```python
from build123d import *

# Parameters (mm, degrees)
SKETCH1_R           = 28
SKETCH1_R_2         = 18
BOSS_EXTRUDE1_DEPTH = 22
SKETCH2_W           = 56
SKETCH2_H           = 56
BOSS_EXTRUDE2_DEPTH = 10
CUT_EXTRUDE1_DEPTH  = 14
SKETCH4_R           = 5
CUT_EXTRUDE2_DEPTH  = 14
SKETCH5_R           = 21.225012464
SKETCH5_R_2         = 11
BOSS_EXTRUDE3_DEPTH = 8
SKETCH6_R           = 50.391738165
CUT_EXTRUDE3_DEPTH  = 14
SKETCH9_R           = 10
CUT_EXTRUDE6_DEPTH  = 10


with BuildPart() as part:
    # Sketch1 → Boss-Extrude1 (new body)
    with BuildSketch(Plane.XY):
        Circle(SKETCH1_R)
        Circle(SKETCH1_R_2, mode=Mode.SUBTRACT)
    extrude(amount=BOSS_EXTRUDE1_DEPTH)

    # Sketch2 → Boss-Extrude2 (add)
    with BuildSketch(Plane.XY.offset(22)):
        Rectangle(SKETCH2_W, SKETCH2_H)
    extrude(amount=BOSS_EXTRUDE2_DEPTH)

    # Sketch3 → Cut-Extrude1 (cut)
    with BuildSketch(Plane(origin=(0, 0, 0), x_dir=(-1, 0, 0), z_dir=(0, 0, -1))):
        Polygon((0, 0), (-28, -28), (28, -28), align=None)
    extrude(amount=-CUT_EXTRUDE1_DEPTH, mode=Mode.SUBTRACT)

    # Sketch4 → Cut-Extrude2 (cut)
    with BuildSketch(Plane(origin=(0, 0, 22), x_dir=(-1, 0, 0), z_dir=(0, 0, -1))):
        Circle(SKETCH4_R)
    extrude(amount=-CUT_EXTRUDE2_DEPTH, mode=Mode.SUBTRACT)

    # Sketch5 → Boss-Extrude3 (add)
    with BuildSketch(Plane(origin=(0, 0, 22), x_dir=(-1, 0, 0), z_dir=(0, 0, -1))):
        Circle(SKETCH5_R)
        Circle(SKETCH5_R_2, mode=Mode.SUBTRACT)
    extrude(amount=BOSS_EXTRUDE3_DEPTH)

    # Sketch6 → Cut-Extrude3 (cut)
    with BuildSketch(Plane(origin=(0, 0, 0), x_dir=(-1, 0, 0), z_dir=(0, 0, -1))):
        Circle(SKETCH6_R)
    extrude(amount=-CUT_EXTRUDE3_DEPTH, mode=Mode.SUBTRACT)

    # Sketch9 → Cut-Extrude6 (cut)
    with BuildSketch(Plane.XY.offset(32)):
        Circle(SKETCH9_R)
    extrude(amount=-CUT_EXTRUDE6_DEPTH, mode=Mode.SUBTRACT)


solid = part.part
```
Geometry: final body of the model. Coordinates: model frame, mm. A direction names the side the tool comes from. Give positions to 0.01 mm unless a question says otherwise; leave off trailing zeros. Order: outer loops, then holes, each group sorted by start corner. A loop starts at its lowest first (then second) coordinate and runs counter-clockwise, first axis right, second up. Notation, with made-up numbers: (4.5, 44) -> (46.5, 44) arc R31 ccw to (46.5, 68) -> close; hole circle Ø4 at (83, -33). An arc over 180 degrees is marked (long way). Write each question's results on one line, items separated by ' | '. Start each with the question number.
1) Section C-C (x = -21). Return loops of the section in (y, z).
2) First-contact query: pin 1 (12 mm diameter, centred on x = 0, y = 0, fed in from -Z). Flat tip, straight axial feed; report the tip coordinate or a pass-through.
3) Section A-A (z = 26). Return loops of the section in (x, y).
4) Line query: line 1 (Y direction, x = 0, z = 24.25); line 2 (Y direction, x = 0, z = 17.25); line 3 (X direction, y = -4.5, z = 28.25). Output: solid intervals per line, ascending. Write a range as from..to.
5) Draft query along X for faces 5 (the cylindrical face through (25.865, -10.724, 17.944)), 6 (the flat face through (21, 22, 22)), 7 (the cylindrical face through (-2.17, -9.76, 27.07)). Return one class per face: pulls with the +X half, pulls with the -X half, needs draft (parallel to the pull), parting line crosses it, or undercut.
6) Set-up query: faces 1 (the flat face through (-22, 21, 22)), 2 (the flat face through (22, -22, 22)), 3 (the flat face through (-22, -21, 22)), 4 (the cylindrical face through (2.38, -10.74, 18.06)). Return all of +Z, -Z, +X, -X, +Y, -Y with unobstructed straight access to the full face (end or side cutting, diameter ignored); none if empty.
Calculated:
1) outline: (-28, 22) -> (-18.52, 22) -> (-18.52, 14) -> (18.52, 14) -> (18.52, 22) -> (28, 22) -> (28, 32) -> (-28, 32) -> close
2) pin 1: through
3) outline: (-28, -28) -> (28, -28) -> (28, 28) -> (-28, 28) -> close; hole circle Ø20 at (0, 0)
4) line 1: -28..-10, 10..28 | line 2: -28..-11, 11..28 | line 3: -28..-8.93, 8.93..28
5) face 5: parting line crosses it | face 6: needs draft | face 7: undercut
6) face 1: -Z, -X, +Y | face 2: -Z, +X, -Y | face 3: -Z, -X, -Y | face 4: -Z
